```python
from build123d import *

# Parameters (mm, degrees)
SKETCH1_R           = 5
BOSS_EXTRUDE1_DEPTH = 6.35
BOSS_EXTRUDE2_START = -15
SKETCH2_R           = 5
BOSS_EXTRUDE2_DEPTH = 15
LPATTERN1_COUNT     = 2
LPATTERN1_PITCH     = 30
SKETCH2_4_R         = 2.5
CUT_EXTRUDE2_DEPTH  = 83.80956065


with BuildPart() as part:
    # Sketch1 → Boss-Extrude1 (new body)
    # profile 1 of 3: a face of its own
    with BuildSketch(Plane(origin=(0, 0, 0), x_dir=(1, 0, 0), z_dir=(0, 1, 0))):
        Polygon((-18.75, 0), (0, 0), (18.75, 0), (37.5, 0), (37.5, 25.4), (-37.5, 25.4), (-37.5, 0), align=None)
        with Locations(Location((-15.279173033, 10.349093201, 0), (0, 0, 270))):
            Circle(SKETCH1_R, mode=Mode.SUBTRACT)
        with Locations(Location((18.543836974, 12.56035891, 0), (0, 0, 270))):
            Circle(SKETCH1_R, mode=Mode.SUBTRACT)
    # profile 2 of 3: a face of its own
    with BuildSketch(Plane(origin=(0, 0, 0), x_dir=(1, 0, 0), z_dir=(0, 1, 0))):
        with BuildLine():
            Line((0, -7.7), (0, 0))
            Line((0, 0), (-18.75, 0))
            Line((-18.75, 0), (-37.5, 0))
            Line((-37.5, 0), (-37.5, -25.4))
            Line((-37.5, -25.4), (0, -25.4))
            Line((0, -25.4), (0, -17.7))
            ThreePointArc((0, -17.7), (-5, -12.7), (0, -7.7))
        make_face()
    # profile 3 of 3: a face of its own
    with BuildSketch(Plane(origin=(0, 0, 0), x_dir=(1, 0, 0), z_dir=(0, 1, 0))):
        with BuildLine():
            Line((18.75, 0), (0, 0))
            Line((0, 0), (0, -7.7))
            ThreePointArc((0, -7.7), (3.535533906, -9.164466094), (5, -12.7))
            ThreePointArc((5, -12.7), (3.535533906, -16.235533906), (0, -17.7))
            Line((0, -17.7), (0, -25.4))
            Line((0, -25.4), (37.5, -25.4))
            Line((37.5, -25.4), (37.5, 0))
            Line((37.5, 0), (18.75, 0))
        make_face()
    extrude(amount=BOSS_EXTRUDE1_DEPTH)

    # Sketch2 → Boss-Extrude2 (add)
    with BuildSketch(Plane.ZY.offset(37.5).offset(BOSS_EXTRUDE2_START)):
        with Locations((-27.448482339, 8.398482339)):
            Circle(SKETCH2_R)
    boss_extrude2 = extrude(amount=-BOSS_EXTRUDE2_DEPTH)

    # LPattern1: Boss-Extrude2 ×2
    with Locations(*[(i * LPATTERN1_PITCH, 0, 0) for i in range(1, LPATTERN1_COUNT)]):
        add(boss_extrude2)

    # Sketch2_4 → Cut-Extrude2 (cut, through all)
    with BuildSketch(Plane.ZY.offset(37.5)):
        with Locations((-27.448482339, 8.398482339)):
            Circle(SKETCH2_4_R)
    extrude(amount=-CUT_EXTRUDE2_DEPTH, mode=Mode.SUBTRACT)


solid = part.part
```
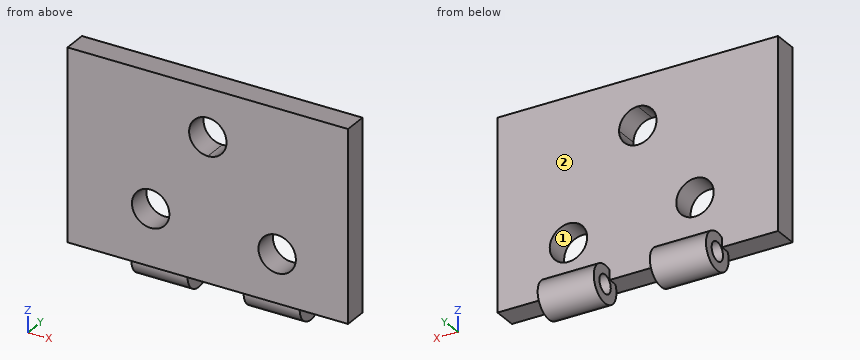
Here's how the part is built. I have some questions about the finished solid (model axes, mm). Face numbers are marked on the shaded views. Round coordinates to 2 decimals unless told otherwise and drop trailing zeros. Order: outer loops, then holes, each group sorted by start corner. A loop starts at its lowest first (then second) coordinate and runs counter-clockwise, first axis right, second up. Notation, with made-up numbers: M 35,39.25 L 71,39.25 A24 cw 71,68.25 Z; hole C 64.5,52 d10. An arc over 180 degrees is marked long. Answer in a Markdown table with one row per item.
Item 1: If I drill on L1, parallel to X at y = 4, z = -25.5; L2, parallel to X at y = 3.75, z = 13; L3, parallel to Z at x = -23, y = 1.25, over which ranges is the centre line in solid material (lowest first)? Write a range as from..to.
A:
| item | result |
|---|---|
| L1 | x = -22.5..-7.5, 7.5..22.5 |
| L2 | x = -37.5..-4.99, 4.99..37.5 |
| L3 | z = -25.4..25.4 |
Item 2: Imagine slicing it at C-C, the plane x = -1. Write out the boundary of the cut face in (y, z), and give its area (3 significant figures).
A:
| item | result |
|---|---|
| outline | M 0,-25.4 L 6.35,-25.4 L 6.35,7.8 L 0,7.8 Z; M 0,17.6 L 6.35,17.6 L 6.35,25.4 L 0,25.4 Z |
| area | 260 mm2 |
Item 3: Imagine slicing it at D-D, the plane y = 1.75. Write out the boundary of the cut face in (x, z).
A:
| item | result |
|---|---|
| outline | M -37.5,-25.4 L 37.5,-25.4 L 37.5,25.4 L -37.5,25.4 Z; hole C -15.28,-10.35 d10; hole C 0,12.7 d10; hole C 18.54,-12.56 d10 |
Item 4: I'm going to push flat-ended pins straight in: pin 1 (1.5 mm diameter, centred on x = -1.5, z = 5.5, fed in from -Y); pin 2 (5 mm diameter, centred on x = -27, z = -23.5, fed in from +Y); pin 3 (6 mm diameter, centred on x = -4, y = 8, fed in from -Z); pin 4 (5 mm diameter, centred on y = 8.5, z = -28.5, fed in from -X). Where does each tip first touch, or does it pass through?
A:
| item | result |
|---|---|
| pin 1 | stops at y = 0 |
| pin 2 | stops at y = 6.35 |
| pin 3 | stops at z = -25.4 |
| pin 4 | stops at x = -22.5 |
Item 5: Thinking about a two-plate mould opening in Z: for the marked faces 1 and 2, which applies, +Z half, -Z half, draft (parallel to the pull), parting line (faces both ways), or undercut?
A:
| item | result |
|---|---|
| face 1 | undercut |
| face 2 | draft |
Item 6: Imagine slicing it at B-B, the plane y = 7.5. Write out the boundary of the cut face in (x, z).
A:
| item | result |
|---|---|
| outline | M -22.5,-32.37 L -7.5,-32.37 L -7.5,-29.78 L -22.5,-29.78 Z; M -22.5,-25.12 L -7.5,-25.12 L -7.5,-22.53 L -22.5,-22.53 Z; M 7.5,-32.37 L 22.5,-32.37 L 22.5,-29.78 L 7.5,-29.78 Z; M 7.5,-25.12 L 22.5,-25.12 L 22.5,-22.53 L 7.5,-22.53 Z |
Item 7: Imagine slicing it at A-A, the plane x = -13. Write out the boundary of the cut face in (y, z), and give its area (3 significant figures).
A:
| item | result |
|---|---|
| outline | M 0,-25.4 L 3.84,-25.4 A5 ccw long 6.35,-22.89 L 6.35,-14.8 L 0,-14.8 Z; M 0,-5.9 L 6.35,-5.9 L 6.35,25.4 L 0,25.4 Z; hole C 8.4,-27.45 d5 |
| area | 321 mm2 |
